from build123d import *

# Parameters (mm, degrees)
F0_R     = 15
F0_R_2   = 5.75
F1_DEPTH = 6
F2_R     = 15
F2_R_2   = 14
F3_DEPTH = 2
F4_SIZE  = 1


with BuildPart() as f1:
    # F0 (on Top) → F1 (new body)
    with BuildSketch(Plane.XY):
        Circle(F0_R)
        Circle(F0_R_2, mode=Mode.SUBTRACT)
    extrude(amount=F1_DEPTH)

    # F2 (on face) → F3 (cut)
    with BuildSketch(Plane(origin=(0, 0, 0), x_dir=(1, 0, 0), z_dir=(0, 0, -1))):
        Circle(F2_R)
        Circle(F2_R_2, mode=Mode.SUBTRACT)
    extrude(amount=-F3_DEPTH, mode=Mode.SUBTRACT)

    # F4
    f4_edges = [f1.edges().sort_by_distance(p)[0] for p in [
        (-5.75, 0, 6),
    ]]
    chamfer(f4_edges, length=F4_SIZE)


solid = f1.part
Work out the finished part from the listing and answer in its coordinate system (mm). Round coordinates to 2 decimals unless told otherwise and drop trailing zeros. Write each loop counter-clockwise with the first axis right and the second up, starting at its lowest first coordinate (ties: lowest second). Pieces come first, ordered by that corner, then holes. Notation, with made-up numbers: (44.25, 55.5) -> (51.25, 55.5) arc R18 ccw to (51.25, 71.5) -> close; hole circle Ø11 at (44.5, -24.75). An arc over 180 degrees is marked (long way). Answer as CSV lines item,"result". Start each with the question number.
(1) The mould has two halves that part along X. Classify faces 1 (the cylindrical face through (-0.75, 5.7, 2.46)), 2 (the flat face through (3.1, -6.5, 6)), 3 (the cylindrical face through (12.932, 5.362, 0.986)): +X half, -X half, draft (parallel to the pull), parting line (faces both ways), or undercut.
(2) Find the intervals of material crossed by probe 1 along Y at (x, z) = (0, 3.05); probe 2 along Y at (x, z) = (0, 1.7); probe 3 along X at (y, z) = (-5.25, 2.45), in increasing order.
(3) The part is cut by section D-D, the plane x = -9. Give the vertices of the cut face in (y, z).
(4) The part is cut by section C-C, the plane z = 1.55. Give the vertices of the cut face in (x, y).
(5) This flat-tipped pin is pushed along its axis until it touches: pin 1 (1 mm diameter, centred on y = -5, z = 1, fed in from +X). Where does it stop, or does it pass through?
(6) The part is cut by section A-A, the plane x = 0. Give the vertices of the cut face in (y, z), then the cut area to 3 significant figures.
Output values:
1,face 1,"undercut"
1,face 2,"draft"
1,face 3,"parting line"
2,probe 1,"y = -15 to -5.75, 5.75 to 15"
2,probe 2,"y = -14 to -5.75, 5.75 to 14"
2,probe 3,"x = -14.05 to -2.35, 2.35 to 14.05"
3,outline,"(-12, 2) -> (-10.72, 2) -> (-10.72, 0) -> (10.72, 0) -> (10.72, 2) -> (12, 2) -> (12, 6) -> (-12, 6) -> close"
4,outline,"circle Ø28 at (0, 0); hole circle Ø11.5 at (0, 0)"
5,pin 1,"stops at x = 13.26"
6,outline,"(-15, 2) -> (-14, 2) -> (-14, 0) -> (-5.75, 0) -> (-5.75, 5) -> (-6.75, 6) -> (-15, 6) -> close; (5.75, 0) -> (14, 0) -> (14, 2) -> (15, 2) -> (15, 6) -> (6.75, 6) -> (5.75, 5) -> close"
6,area,"106 mm²"
